Autodesk Inventor part; units mm, degrees
ref_plane "YZ Plane" through (0, 0, 0) normal (1, 0, 0) x (0, 1, 0)
ref_plane "XZ Plane" through (0, 0, 0) normal (0, 1, 0) x (-1, 0, 0)
ref_plane "XY Plane" through (0, 0, 0) normal (0, 0, 1) x (1, 0, 0)
sketch "Skizze1" plane through (0, 0, 0) normal (0, 0, 1) x (1, 0, 0)
  circle A0 centre (0, 0) radius 4.5
  dimension "d0" = 9
extrude "Extrusion1" add sketch "Skizze1" along normal blind 11
sketch "Skizze2" plane through (0, 0, 11) normal (0, 0, 1) x (1, 0, 0)
  circle A0 centre (0, 0) radius 2.5
  dimension "d3" = 5
extrude "Extrusion2" cut sketch "Skizze2" against normal blind 11
sketch "Skizze5" plane through (0, 0, 0) normal (0, 1, 0) x (-1, 0, 0)
  line L0 (4.5, 11) -> (-4.5, 11)
  line L1 (-4.5, 0) -> (4.5, 0)
  line L2 (4.5, 0) -> (4.5, 11)
  line L3 (-4.5, 0) -> (-4.5, 11)
  arc A0 (4.5, 10) -> (4.5, 3.1436) centre (10, 6.5718) ccw
  line L4 (4.5, 11) -> (-4.5, 11)
  line L5 (3.5, 11) -> (3.5, 0)
  line L6 (-4.5, 0) -> (4.5, 0)
  line L7 (4.5, 3.1436) -> (4.5, 10)
  line L8 (0, -2.2) -> (0, 13.2)
  point P0 (0, 0)
  dimension "d12" = 1
  dimension "d13" = 5.5
revolve "Umdrehung1" cut sketch "Skizze5" angle 360 about axis through (0, 0, -10) along (0, 0, 1) contours L2 A0
properties part number "MK8_Drive_gear" material "Stahl, Kohlenstoff"
CAD build for the part. Positions are in the model's coordinates, mm. Give positions to 0.01 mm unless a question says otherwise; leave off trailing zeros. Loops run counter-clockwise (first coordinate to the right, second up) from the corner with the lowest first, then second, coordinate; pieces in that order, holes last. Notation, with made-up numbers: M 66,26 L 103,26 A19 ccw 103,41 Z; hole C 57.25,-39.5 d3. An arc over 180 degrees is marked long. One line per question, with ' | ' between items. Start each with the question number.
1. Saw through at D-D on z = 8.25. Give the cut face in (x, y).
2. Saw through at C-C on z = 2.5. Give the cut face in (x, y).
3. Flat gauge pins, fed straight in: pin 1 (4 mm diameter, centred on x = 0, y = 0, fed in from -Z); pin 2 (3 mm diameter, centred on x = 1.5, z = 8, fed in from +Y). Where does each tip first touch, or does it go through?
4. Two-plate mould, pull along X, no slides. Class faces 1 (the face through (2, -2, 0)), 2 (the face through (-0.59, -4.46, 10.49)), 3 (the face through (-0.54, -2.44, 5.58)): pulls with the +X half, pulls with the -X half, needs draft (parallel to the pull), parting line crosses it, or undercut.
5. Saw through at A-A on x = 0. Give the cut face in (y, z).
6. Probe L1, parallel to Y at x = 0, z = 2.5; L2, parallel to X at y = -1.5, z = 3; L3, parallel to X at y = 1.25, z = 10.75. List the from-to ranges inside material, lowest first. Write a range as from..to.
Result sheet:
1) outline: C 0,0 d7.48; hole C 0,0 d5
2) outline: C 0,0 d9; hole C 0,0 d5
3) pin 1: passes through | pin 2: stops at y = 4.06
4) face 1: needs draft | face 2: parting line crosses it | face 3: undercut
5) outline: M -4.5,0 L -2.5,0 L -2.5,11 L -4.5,11 L -4.5,10 A6.48 cw -4.5,3.14 Z; M 2.5,0 L 4.5,0 L 4.5,3.14 A6.48 cw 4.5,10 L 4.5,11 L 2.5,11 Z
6) L1: y = -4.5..-2.5, 2.5..4.5 | L2: x = -4.24..-2, 2..4.24 | L3: x = -4.32..-2.17, 2.17..4.32
